Model file for the job. Use its own axes, mm. A direction names the side the tool comes from. Give positions to 0.01 mm unless a question says otherwise; leave off trailing zeros. Write each loop counter-clockwise with the first axis right and the second up, starting at its lowest first coordinate (ties: lowest second). Pieces come first, ordered by that corner, then holes. Notation, with made-up numbers: (40, -4.75) - (80, -4.75) arc R14 ccw to (80, 16.25) - close; hole circle Ø5 at (-20, 5). An arc over 180 degrees is marked (long way). One line per item, written item: value. Start each with the question number.
(1) Cut at D-D, the plane y = -13. List the corners of the cut face in (x, z), and give its area (3 significant figures).
(2) Cut at B-B, the plane x = -104. List the corners of the cut face in (y, z).
(3) Cut at A-A, the plane z = -37.5. List the corners of the cut face in (x, y).
(4) Mould opens along Z. For faces 1 (the face through (-92.938, 22.446, -12.305)), 2 (the face through (-107, -10, -147)), 3 (the face through (-93, 25.959, -134)) say: pulls with the +Z half, pulls with the -Z half, needs draft (parallel to the pull), parting line crosses it, or undercut.
(5) Drop flat-ended pins along their axis: P1, Ø9, axis at y = -41.5, z = -138, coming from the -X side; P2, Ø1.8, axis at y = 20.96, z = -134.5, coming from the -X side; P3, Ø4.5, axis at x = -100.5, z = -107.5, coming from the -Y side; P4, Ø3.5, axis at y = 20.96, z = -12.5, coming from the -X side. Give the stop position or say it passes through.
(6) 3-axis set-ups, long thin cutter, end or side, ignore diameter. For faces 4 (the face through (-94.459, 22, -25)), 5 (the face through (-93, -41, -50)), 6 (the face through (-94.459, -42, -25)), 7 (the face through (-93, 21, -50)): which of +Z, -Z, +X, -X, +Y, -Y reach the whole face in a straight line?
(7) Cut at C-C, the plane z = -67.5. List the corners of the cut face in (x, y), and give its area (3 significant figures).
(8) Probe L1, parallel to Y at x = -93.2, z = -12.5; L2, parallel to Y at x = -93.7, z = -12.5 (3 decimals); L3, parallel to Y at x = -101.25, z = -16.5. List the from-to ranges inside material, lowest first.
from build123d import *

# Parameters (mm, degrees)
BOSS_EXTRUDE1_DEPTH = 147
SKETCH2_W           = 50
SKETCH2_H           = 10
SKETCH2_R           = 1.5
SKETCH2_W_2         = 25
BOSS_EXTRUDE2_DEPTH = 3
FILLET1_R           = 10
FILLET2_R           = 2


with BuildPart() as part:
    # Sketch1 → Boss-Extrude1 (new body)
    with BuildSketch(Plane.XY):
        with BuildLine():
            Line((-91.459491941, 15.958690151), (-116.459491941, 15.958690151))
            Line((-116.459491941, 15.958690151), (-116.459491941, -36.041309849))
            Line((-116.459491941, -36.041309849), (-91.459491941, -36.041309849))
            Line((-91.459491941, -36.041309849), (-91.459491941, -28.371612629))
            ThreePointArc((-91.459491941, -28.371612629), (-105.459491941, -10.041309849), (-91.459491941, 8.288992931))
            Line((-91.459491941, 8.288992931), (-91.459491941, 15.958690151))
        make_face()
    extrude(amount=-BOSS_EXTRUDE1_DEPTH)

    # Sketch2 → Boss-Extrude2 (add)
    # profile 1 of 4: a face of its own
    with BuildSketch(Plane(origin=(-91.459491941, 0, 0), x_dir=(0, 0, -1), z_dir=(1, 0, 0))):
        with Locations((25, 20.958690151)):
            Rectangle(SKETCH2_W, SKETCH2_H)
        with Locations((12.5, 20.958690151)):
            Circle(SKETCH2_R, mode=Mode.SUBTRACT)
        with Locations(Location((37.5, 20.958690151, 0), (0, 0, 180))):
            Circle(SKETCH2_R, mode=Mode.SUBTRACT)
    # profile 2 of 4: a face of its own
    with BuildSketch(Plane(origin=(-91.459491941, 0, 0), x_dir=(0, 0, -1), z_dir=(1, 0, 0))):
        with Locations((134.5, 20.958690151)):
            Rectangle(SKETCH2_W_2, SKETCH2_H)
        with Locations((134.5, 20.958690151)):
            Circle(SKETCH2_R, mode=Mode.SUBTRACT)
    # profile 3 of 4: a face of its own
    with BuildSketch(Plane(origin=(-91.459491941, 0, 0), x_dir=(0, 0, -1), z_dir=(1, 0, 0))):
        with Locations((25, -41.041309849)):
            Rectangle(SKETCH2_W, SKETCH2_H)
        with Locations((37.5, -41.041309849)):
            Circle(SKETCH2_R, mode=Mode.SUBTRACT)
        with Locations(Location((12.5, -41.041309849, 0), (0, 0, 180))):
            Circle(SKETCH2_R, mode=Mode.SUBTRACT)
    # profile 4 of 4: a face of its own
    with BuildSketch(Plane(origin=(-91.459491941, 0, 0), x_dir=(0, 0, -1), z_dir=(1, 0, 0))):
        with Locations((134.5, -41.041309849)):
            Rectangle(SKETCH2_W_2, SKETCH2_H)
        with Locations(Location((134.5, -41.041309849, 0), (0, 0, 180))):
            Circle(SKETCH2_R, mode=Mode.SUBTRACT)
    extrude(amount=-BOSS_EXTRUDE2_DEPTH)

    # Fillet1
    fillet1_edges = [part.edges().sort_by_distance(p)[0] for p in [
        (-116.459491941, 15.958690151, -73.5),
        (-116.459491941, -36.041309849, -73.5),
    ]]
    fillet(fillet1_edges, radius=FILLET1_R)

    # Fillet2
    fillet2_edges = [part.edges().sort_by_distance(p)[0] for p in [
        (-94.459491941, 15.958690151, -25),
        (-94.459491941, 15.958690151, -134.5),
        (-94.459491941, -36.041309849, -25),
        (-94.459491941, -36.041309849, -134.5),
    ]]
    fillet(fillet2_edges, radius=FILLET2_R)


solid = part.part
Answers follow:
1. outline: (-116.46, -147) - (-105.23, -147) - (-105.23, 0) - (-116.46, 0) - close
1. area: 1,650 mm²
2. outline: (-36.04, -147) - (-17.34, -147) - (-17.34, 0) - (-36.04, 0) - close; (-2.74, -147) - (15.96, -147) - (15.96, 0) - (-2.74, 0) - close
3. outline: (-116.46, -26.04) arc R10 ccw to (-106.46, -36.04) - (-96.46, -36.04) arc R2 cw to (-94.46, -38.04) - (-94.46, -39.54) - (-91.46, -39.54) - (-91.46, -28.37) arc R19 cw to (-91.46, 8.29) - (-91.46, 19.46) - (-94.46, 19.46) - (-94.46, 17.96) arc R2 cw to (-96.46, 15.96) - (-106.46, 15.96) arc R10 ccw to (-116.46, 5.96) - close; (-94.46, -46.04) - (-91.46, -46.04) - (-91.46, -42.54) - (-94.46, -42.54) - close; (-94.46, 22.46) - (-91.46, 22.46) - (-91.46, 25.96) - (-94.46, 25.96) - close
4. face 1: undercut
4. face 2: pulls with the -Z half
4. face 3: needs draft
5. P1: stops at x = -94.75
5. P2: passes through
5. P3: stops at y = -36.04
5. P4: stops at x = -94.46
6. face 4: +Z, -Z, -X, +Y
6. face 5: +X, -X, -Y
6. face 6: +Z, -Z, -X, -Y
6. face 7: +X, -X, +Y
7. outline: (-116.46, -26.04) arc R10 ccw to (-106.46, -36.04) - (-91.46, -36.04) - (-91.46, -28.37) arc R19 cw to (-91.46, 8.29) - (-91.46, 15.96) - (-106.46, 15.96) arc R10 ccw to (-116.46, 5.96) - close
7. area: 878 mm²
8. L1: y = -46.04 to -42.54, -39.54 to -27.81, 7.72 to 19.46, 22.46 to 25.96
8. L2: y = -46.041 to -42.541, -39.541 to -27.608, 7.525 to 19.459, 22.459 to 25.959
8. L3: y = -36.04 to -21.97, 1.89 to 15.96
